Drawing for the job (mm, zero at the part's lowest x, y, z). Coordinates: 2 decimals unless noted, no trailing zeros. Order: outer loops, then holes, each group sorted by start corner. A loop starts at its lowest first (then second) coordinate and runs counter-clockwise, first axis right, second up.
1) Pin check, flat tip, straight feed: pin 1 Ø3 at (x, y) = (58, 7.5) entering from -Z. Stop position of the tip, or through.
2) Cut at B-B (y = 3.75). List the corners of the cut face in (x, z).
3) Mould opens along X. For the marked faces 1, 2 and 3 say: +X half, -X half, draft (parallel to the pull), parting line (faces both ways), or undercut.
4) Cut at A-A (x = 36.5). List the corners of the cut face in (y, z), and give its area (3 significant figures).
5) Wall check: L1, parallel to Z at x = 45, y = 4.5; L2, parallel to X at y = 1.5, z = 33; L3, parallel to Y at x = 16.5, z = 111. Give the ranges that are in metal, low to high.
6) Cut at C-C (x = 23.5). List the corners of the cut face in (y, z).
7) Cut at D-D (z = 102.5). List the corners of the cut face in (x, y), and give its area (3 significant figures).
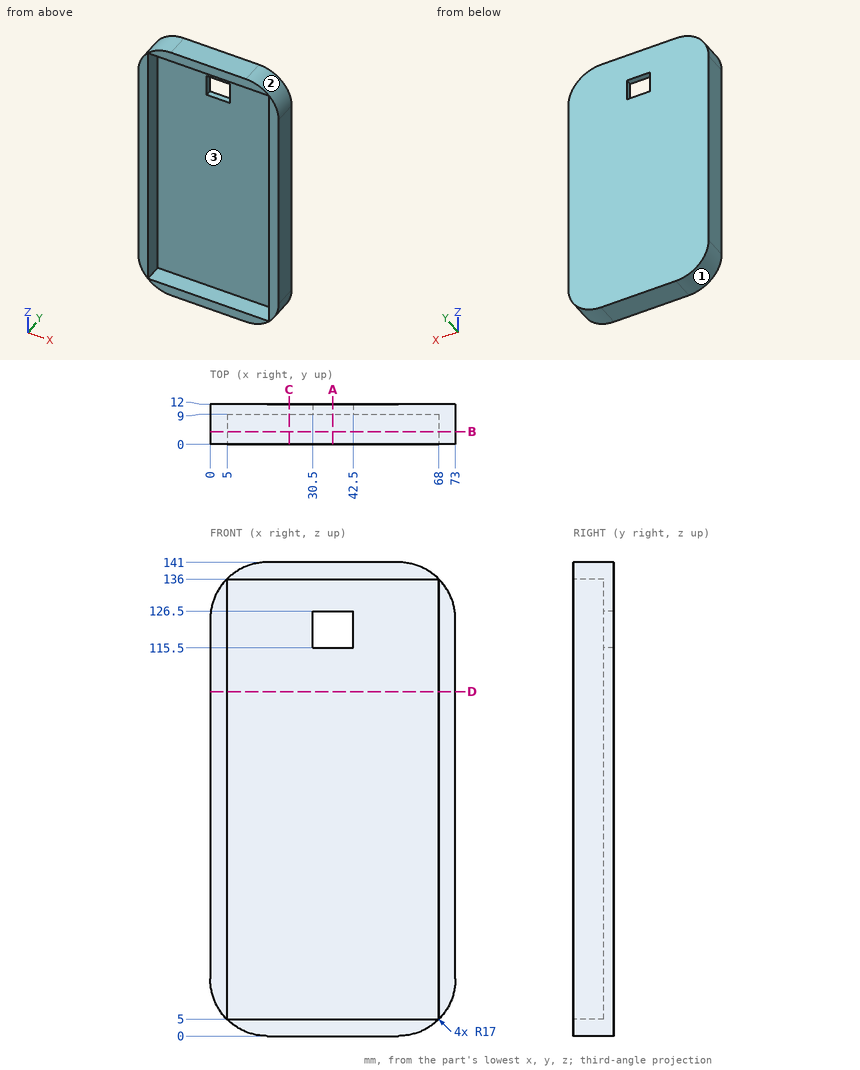
Geometry check:
1. pin 1: stops at z = 0.01
2. outline: (0, 17) arc R17 ccw to (17, 0) - (56, 0) arc R17 ccw to (73, 17) - (73, 124) arc R17 ccw to (56, 141) - (17, 141) arc R17 ccw to (0, 124) - close; hole (5, 5) - (68, 5) - (68, 136) - (5, 136) - close
3. face 1: -X half
3. face 2: +X half
3. face 3: undercut
4. outline: (0, 0) - (12, 0) - (12, 115.5) - (9, 115.5) - (9, 5) - (0, 5) - close; (0, 136) - (9, 136) - (9, 126.5) - (12, 126.5) - (12, 141) - (0, 141) - close
4. area: 480 mm2
5. L1: z = 0 to 5, 136 to 141
5. L2: x = 0 to 5, 68 to 73
5. L3: y = 9 to 12
6. outline: (0, 0) - (12, 0) - (12, 141) - (0, 141) - (0, 136) - (9, 136) - (9, 5) - (0, 5) - close
7. outline: (0, 0) - (5, 0) - (5, 9) - (68, 9) - (68, 0) - (73, 0) - (73, 12) - (0, 12) - close
7. area: 309 mm2
